from build123d import *

# Parameters (mm, degrees)
F0_W     = 609.6
F0_H     = 25.4
F1_DEPTH = 25.4
F2_W     = 20.32
F2_H     = 20.32
F3_DEPTH = 609.6
F4_R     = 2.5527
F5_DEPTH = 25.4


with BuildPart() as f1:
    # F0 (on Front) → F1 (new body)
    with BuildSketch(Plane.XZ):
        with Locations((209.717386, 30.944633)):
            Rectangle(F0_W, F0_H)
    extrude(amount=F1_DEPTH)

    # F2 (on face) → F3 (cut)
    with BuildSketch(Plane(origin=(-95.082614, 0, 0), x_dir=(0, -1, 0), z_dir=(-1, 0, 0))):
        with Locations((12.7, 30.944633)):
            Rectangle(F2_W, F2_H)
    extrude(amount=-F3_DEPTH, mode=Mode.SUBTRACT)

    # F4 (on face) → F5 (cut)
    with BuildSketch(Plane.XZ.offset(25.4)):
        with Locations((501.817386, 30.944633)):
            Circle(F4_R)
        with Locations((476.417386, 30.944633)):
            Circle(F4_R)
        with Locations((-82.382614, 30.944633)):
            Circle(F4_R)
        with Locations((-31.582614, 30.944633)):
            Circle(F4_R)
    extrude(amount=-F5_DEPTH, mode=Mode.SUBTRACT)


solid = f1.part
Build history of the part. All positions in model axes, mm. A direction names the side the tool comes from. Coordinates: 2 decimals unless noted, no trailing zeros. Order: outer loops, then holes, each group sorted by start corner. A loop starts at its lowest first (then second) coordinate and runs counter-clockwise, first axis right, second up. Notation, with made-up numbers: (-2, 10) - (17, 10) arc R25 cw to (17, 22) - close; hole circle Ø1 at (67, 77). An arc over 180 degrees is marked (long way). Put each result on its own line as item: value.
1. Pull direction Y, two halves, no side cores. Call faces 3 (the face through (205, 0, 31)), 4 (the face through (205, -13, 18.245)), 5 (the face through (205, -13, 20.785)): pulls with the +Y half, pulls with the -Y half, needs draft (parallel to the pull), parting line crosses it, or undercut.
Answer sheet:
face 3: pulls with the +Y half
face 4: needs draft
face 5: undercut
2. Tool access for faces 1 (the face through (514.517, -13, 42)), 2 (the face through (205, -22.86, 31)): list every direction of +Z, -Z, +X, -X, +Y, -Y with a clear straight run to the whole face (end or side of a thin tool).
Answer sheet:
face 1: +Z, -Z, +X, +Y, -Y
face 2: +X, -X
3. Drop a flat-ended pin along its axis: P1, Ø8, axis at x = -82.38, z = 30.94, coming from the +Y side. Give the stop position or say it passes through.
Answer sheet:
P1: stops at y = 0
4. Saw through at A-A (y = -16.25). Write the cut outline in (x, z), and give its area (3 significant figures).
Answer sheet:
outline: (-95.08, 18.24) - (514.52, 18.24) - (514.52, 20.78) - (-95.08, 20.78) - close; (-95.08, 41.1) - (514.52, 41.1) - (514.52, 43.64) - (-95.08, 43.64) - close
area: 3,100 mm^2
5. Probe line 1 along Y through (x, z) = (-11, 21.25); line 2 along Z through (x, y) = (15, -8.25). List the from-to ranges inside material, lowest first. Write a range as [from, to].
Answer sheet:
line 1: y = [-25.4, -22.86], [-2.54, 0]
line 2: z = [18.24, 20.78], [41.1, 43.64]
6. Saw through at B-B (x = -3). Write the cut outline in (y, z).
Answer sheet:
outline: (-25.4, 18.24) - (0, 18.24) - (0, 43.64) - (-25.4, 43.64) - close; hole (-22.86, 20.78) - (-2.54, 20.78) - (-2.54, 41.1) - (-22.86, 41.1) - close
